from build123d import *

# Parameters (mm, degrees)
SKETCH1_W           = 83
SKETCH1_H           = 59
BOSS_EXTRUDE1_DEPTH = 3
SKETCH2_W           = 83
SKETCH2_H           = 59
BOSS_EXTRUDE2_DEPTH = 4


with BuildPart() as part:
    # Sketch1 → Boss-Extrude1 (new body)
    with BuildSketch(Plane(origin=(0, 0, 0), x_dir=(1, 0, 0), z_dir=(0, 1, 0))):
        with Locations((41.5, 29.5)):
            Rectangle(SKETCH1_W, SKETCH1_H)
    extrude(amount=BOSS_EXTRUDE1_DEPTH)

    # Sketch2 → Boss-Extrude2 (add)
    with BuildSketch(Plane(origin=(0, 3, 0), x_dir=(1, 0, 0), z_dir=(0, 1, 0))):
        with Locations((41.5, 29.5)):
            Rectangle(SKETCH2_W, SKETCH2_H)
        with BuildLine():
            Line((3, 46.5), (3, 12.5))
            ThreePointArc((3, 12.5), (9.717514421, 9.717514421), (12.5, 3))
            Line((12.5, 3), (70.5, 3))
            ThreePointArc((70.5, 3), (73.282485579, 9.717514421), (80, 12.5))
            Line((80, 12.5), (80, 46.5))
            ThreePointArc((80, 46.5), (73.282485579, 49.282485579), (70.5, 56))
            Line((70.5, 56), (12.5, 56))
            ThreePointArc((12.5, 56), (9.717514421, 49.282485579), (3, 46.5))
        make_face(mode=Mode.SUBTRACT)
    extrude(amount=BOSS_EXTRUDE2_DEPTH)


solid = part.part
The listing builds one solid part. Answer for the finished solid, in the listing's coordinates (mm). A direction names the side the tool comes from. Round coordinates to 2 decimals unless told otherwise and drop trailing zeros. Order: outer loops, then holes, each group sorted by start corner. A loop starts at its lowest first (then second) coordinate and runs counter-clockwise, first axis right, second up. Notation, with made-up numbers: (-20, 76.5) -> (-3, 76.5) arc R21 cw to (-3, 109.5) -> close; hole circle Ø1 at (4.25, -23). An arc over 180 degrees is marked (long way). Write each question's results on one line, items separated by ' | '. Start each with the question number.
Q1. Which of the six approach directions +Z, -Z, +X, -X, +Y, -Y give full straight-line access (tool end or side, diameter ignored) to faces 4 (the flat face through (41, 0, -30)), 5 (the flat face through (80, 5, -29))?
Q2. Straight lines are drawn through the part: probe 1 along X at (y, z) = (4.25, -41); probe 2 along Z at (x, y) = (39, 4.25); probe 3 along Y at (x, z) = (31.5, -45.5). For each, find the intervals that lie inside material, in ascending order. Write a range as from..to.
Q3. Find section A-A (y = 4.5). Determine the outline of the cut face in (x, z).
Q4. The mould has two halves that part along Z. Classify faces 1 (the flat face through (83, 3, -29)), 2 (the flat face through (42, 5, -56)), 3 (the flat face through (41, 3, 0)): pulls with the +Z half, pulls with the -Z half, needs draft (parallel to the pull), parting line crosses it, or undercut.
Q5. Each of these flat-tipped pins is pushed along its axis until it touches: pin 1 (16 mm diameter, centred on x = 51.5, z = -41.5, fed in from +Y); pin 2 (1.5 mm diameter, centred on x = 74, z = -8, fed in from -Y). Where does it stop, or does it pass through?
Q6. Find section C-C (z = -14). Determine the outline of the cut face in (x, y), then the cut area to 3 significant figures.
Q7. Find section B-B (x = 64). Determine the outline of the cut face in (y, z), then the cut area to 3 significant figures.
Worked answers:
1) face 4: +Z, -Z, +X, -X, -Y | face 5: +Y
2) probe 1: x = 0..3, 80..83 | probe 2: z = -59..-56, -3..0 | probe 3: y = 0..3
3) outline: (0, -59) -> (83, -59) -> (83, 0) -> (0, 0) -> close; hole (3, -46.5) arc R9.5 cw to (12.5, -56) -> (70.5, -56) arc R9.5 cw to (80, -46.5) -> (80, -12.5) arc R9.5 cw to (70.5, -3) -> (12.5, -3) arc R9.5 cw to (3, -12.5) -> close
4) face 1: needs draft | face 2: undercut | face 3: pulls with the +Z half
5) pin 1: stops at y = 3 | pin 2: stops at y = 0
6) outline: (0, 0) -> (83, 0) -> (83, 7) -> (80, 7) -> (80, 3) -> (3, 3) -> (3, 7) -> (0, 7) -> close | area: 273 mm2
7) outline: (0, -59) -> (7, -59) -> (7, -56) -> (3, -56) -> (3, -3) -> (7, -3) -> (7, 0) -> (0, 0) -> close | area: 201 mm2
